Autodesk Inventor part; units mm, degrees
ref_plane "YZ Plane" through (0, 0, 0) normal (1, 0, 0) x (0, 1, 0)
ref_plane "XZ Plane" through (0, 0, 0) normal (0, 1, 0) x (-1, 0, 0)
ref_plane "XY Plane" through (0, 0, 0) normal (0, 0, 1) x (1, 0, 0)
sketch "Sketch1" plane through (0, 0, 0) normal (0, 0, 1) x (1, 0, 0)
  line L0 (0, 8.6995) -> (0, 0)
  line L1 (0, 0) -> (2.8194, 0)
  line L2 (2.8194, 0) -> (2.7559, 1.1684)
  line L3 (2.7559, 1.1684) -> (2.4384, 1.1684)
  line L4 (2.4384, 1.1684) -> (2.4384, 6.2611)
  arc A0 (2.4384, 6.2611) -> (0, 8.6995) centre (0, 6.2611) ccw
  dimension "d0" = 2.4384
  dimension "d1" = 2.8194
  dimension "d2" = 2.7559
  dimension "d3" = 1.1684
  dimension "d4" = 8.6995
revolve "Revolution1" add sketch "Sketch1" angle 360 about axis through (0, 8.6995, 0) along (0, -1, 0)
sketch "Sketch2" plane through (0, 0, 0) normal (0, -1, 0) x (1, 0, 0)
  line L0 (0.235, 2.1273) -> (-0.2349, 2.1273)
  line L1 (-0.2349, 2.1273) -> (-0.2349, 1.4034)
  line L2 (-0.2349, 1.4034) -> (0.235, 1.4034)
  line L3 (0.235, 1.4034) -> (0.235, 2.1273)
  line L4 (0.235, 2.1273) -> (-0.2349, 1.4034) construction
  line L5 (-0.2349, 2.1273) -> (0.235, 1.4034) construction
  line L6 (0.235, 0.9504) -> (-0.2349, 0.9504)
  line L7 (-0.2349, 0.9504) -> (-0.2349, 0.2265)
  line L8 (-0.2349, 0.2265) -> (0.235, 0.2265)
  line L9 (0.235, 0.2265) -> (0.235, 0.9504)
  line L10 (0.235, 0.9504) -> (-0.2349, 0.2265) construction
  line L11 (-0.2349, 0.9504) -> (0.235, 0.2265) construction
  line L12 (0.235, -0.2265) -> (-0.2349, -0.2265)
  line L13 (-0.2349, -0.2265) -> (-0.2349, -0.9504)
  line L14 (-0.2349, -0.9504) -> (0.235, -0.9504)
  line L15 (0.235, -0.9504) -> (0.235, -0.2265)
  line L16 (0.235, -0.2265) -> (-0.2349, -0.9504) construction
  line L17 (-0.2349, -0.2265) -> (0.235, -0.9504) construction
  line L18 (0.2349, -1.4033) -> (-0.2349, -1.4033)
  line L19 (-0.2349, -1.4033) -> (-0.2349, -2.1273)
  line L20 (-0.2349, -2.1273) -> (0.2349, -2.1273)
  line L21 (0.2349, -2.1273) -> (0.2349, -1.4033)
  line L22 (0.2349, -1.4033) -> (-0.2349, -2.1273) construction
  line L23 (-0.2349, -1.4033) -> (0.2349, -2.1273) construction
  circle A0 centre (0, 0) radius 2.7559 construction
  line L24 (2.7559, 0) -> (-2.7559, 0) construction
  point P0 (0, 0)
  point P1 (0, 1.7653)
  point P2 (0, 0.5884)
  point P3 (0, -0.5884)
  point P4 (0, -1.7653)
  point P5 (0, -1.7653)
  point P6 (0, -0.9504)
  point P7 (0, -0.5884)
  point P8 (0, 0.5884)
  point P9 (0, 0.2265)
  point P10 (0, 1.7653)
  point P11 (0, -0.5884)
  dimension "d6" = 0.4699
  dimension "d7" = 0.7239
  dimension "d8" = 4.2545
  dimension "d9" = 0.453
  dimension "d10" = 0.453
extrude "Extrusion1" add sketch "Sketch2" along normal blind 24.7396
sketch "Sketch3" plane through (0, -24.7396, 0) normal (0, -1, 0) x (1, 0, 0)
  line L0 (0.235, 2.1273) -> (-0.2349, 2.1273)
  line L1 (-0.2349, 2.1273) -> (-0.2349, 1.4034)
  line L2 (-0.2349, 1.4034) -> (0.235, 1.4034)
  line L3 (0.235, 1.4034) -> (0.235, 2.1273)
  line L4 (0.235, -0.2265) -> (-0.2349, -0.2265)
  line L5 (-0.2349, -0.2265) -> (-0.2349, -0.9504)
  line L6 (-0.2349, -0.9504) -> (0.235, -0.9504)
  line L7 (0.235, -0.9504) -> (0.235, -0.2265)
  point P0 (0, 0)
extrude "Extrusion2" add sketch "Sketch3" along normal blind 1.2065
sketch "Sketch4" plane through (0, -24.7396, 0) normal (0, -1, 0) x (1, 0, 0)
  line L0 (0.235, 0.9504) -> (-0.2349, 0.9504)
  line L1 (-0.2349, 0.9504) -> (-0.2349, 0.2265)
  line L2 (-0.2349, 0.2265) -> (0.235, 0.2265)
  line L3 (0.235, 0.2265) -> (0.235, 0.9504)
  point P0 (0, 0)
extrude "Extrusion3" add sketch "Sketch4" along normal blind 2.0193
sketch "Sketch5" plane through (0, -26.7589, 0) normal (0, -1, 0) x (1, 0, 0)
  line L0 (0.235, -0.2265) -> (0.235, -0.9504)
  line L1 (0.235, -0.9504) -> (-0.2349, -0.9504)
  line L2 (-0.2349, -0.9504) -> (-0.2349, -0.2265)
  line L3 (-0.2349, -0.2265) -> (0.235, -0.2265)
  line L4 (0.235, 2.1273) -> (0.235, 1.4034)
  line L5 (0.235, 1.4034) -> (-0.2349, 1.4034)
  line L6 (-0.2349, 1.4034) -> (-0.2349, 2.1273)
  line L7 (-0.2349, 2.1273) -> (0.235, 2.1273)
  line L8 (0.235, 0.9504) -> (0.235, 0.2265)
  line L9 (0.235, 0.2265) -> (-0.2349, 0.2265)
  line L10 (-0.2349, 0.2265) -> (-0.2349, 0.9504)
  line L11 (-0.2349, 0.9504) -> (0.235, 0.9504)
  line L12 (0.2349, -1.4033) -> (0.2349, -2.1273)
  line L13 (0.2349, -2.1273) -> (-0.2349, -2.1273)
  line L14 (-0.2349, -2.1273) -> (-0.2349, -1.4033)
  line L15 (-0.2349, -1.4033) -> (0.2349, -1.4033)
  circle A0 centre (0, 0) radius 2.8194
  circle A1 centre (0, 1.7653) radius 0.127
  circle A2 centre (0, 0.5884) radius 0.127
  circle A3 centre (0, -0.5884) radius 0.127
  circle A4 centre (0, -1.7653) radius 0.127
  point P0 (0.235, 1.7653)
  point P1 (0.235, 0.5884)
  point P2 (0.235, -0.5884)
  point P3 (0.2349, -1.7653)
  point P4 (0, 1.4034)
  dimension "d17" = 0.254
extrude "Extrusion4" cut sketch "Sketch5" against normal blind 6.35 contours A1 | A2 | A3 | A4
equation "\"d9\" = d10"
properties part number "Clipped LED"
The listing builds one solid part. Answer for the finished solid, in the listing's coordinates (mm). Round coordinates to 2 decimals unless told otherwise and drop trailing zeros. Write each loop counter-clockwise with the first axis right and the second up, starting at its lowest first coordinate (ties: lowest second). Pieces come first, ordered by that corner, then holes. Notation, with made-up numbers: (9, 20.5) - (68, 20.5) arc R27 cw to (68, 52.5) - close; hole circle Ø4 at (12, 31.25). An arc over 180 degrees is marked (long way). Use one line per item in the form item = value. Start each with the question number.
Item 1: Find the intervals of material crossed by line 1 (X direction, y = -6.5, z = 0.6) (3 decimals); line 2 (Y direction, x = -0.55, z = 1.9); line 3 (X direction, y = 6, z = 2.05), in increasing order. Write a range as [from, to].
Item 2: A cutting plane is placed at A-A (y = -7). Write down the section's boundary in (x, z) (1 decimal), plus the area to 3 significant figures.
Item 3: Flat-ended cylindrical pins translate along their axes: pin 1 Ø1.5 at (x, y) = (0, -15.5) entering from -Z; pin 2 Ø0.8 at (y, z) = (-14.5, -2) entering from -X; pin 3 Ø0.8 at (y, z) = (-10, 1) entering from +X (3 decimals). Find the tip coordinate at first contact, or state that the pin passes through.
The answers:
q1.line_1 = [-0.235, 0.235]
q1.line_2 = [0, 7.69]
q1.line_3 = [-1.32, 1.32]
q2.outline = (-0.2, -2.1) - (0.2, -2.1) - (0.2, -1.4) - (-0.2, -1.4) - close; (-0.2, -1) - (0.2, -1) - (0.2, -0.2) - (-0.2, -0.2) - close; (-0.2, 0.2) - (0.2, 0.2) - (0.2, 1) - (-0.2, 1) - close; (-0.2, 1.4) - (0.2, 1.4) - (0.2, 2.1) - (-0.2, 2.1) - close
q2.area = 1.36 mm^2
q3.pin_1 = -2.13
q3.pin_2 = -0.23
q3.pin_3 = 0.235
